The listing builds one solid part. Answer for the finished solid, in the listing's coordinates (mm). Face numbers are marked on the shaded views. A direction names the side the tool comes from. Coordinates: 2 decimals unless noted, no trailing zeros. Write each loop counter-clockwise with the first axis right and the second up, starting at its lowest first coordinate (ties: lowest second). Pieces come first, ordered by that corner, then holes. Notation, with made-up numbers: M -1,-29.75 L 58,-29.75 A17 ccw 58,-19.75 Z; hole C -7.75,34 d5. An arc over 180 degrees is marked long. Answer as CSV lines item,"result". Start each with the question number.
```python
from build123d import *

# Parameters (mm, degrees)
SKETCH1_W           = 60
SKETCH1_H           = 24
BOSS_EXTRUDE1_DEPTH = 3.3
SKETCH2_W           = 3.3
SKETCH2_H           = 24
BOSS_EXTRUDE2_DEPTH = 61.3
SKETCH7_R           = 1.5
SKETCH7_W           = 29.4
SKETCH7_H           = 14
CUT_EXTRUDE4_DEPTH  = 3.3
SKETCH9_W           = 14
SKETCH9_H           = 28
CUT_EXTRUDE5_DEPTH  = 10


with BuildPart() as part:
    # Sketch1 → Boss-Extrude1 (new body)
    with BuildSketch(Plane(origin=(0, 0, 0), x_dir=(1, 0, 0), z_dir=(0, 1, 0))):
        Rectangle(SKETCH1_W, SKETCH1_H)
    extrude(amount=BOSS_EXTRUDE1_DEPTH)

    # Sketch2 → Boss-Extrude2 (add)
    with BuildSketch(Plane(origin=(0, 0, 0), x_dir=(1, 0, 0), z_dir=(0, 1, 0))):
        with Locations((-28.35, 0)):
            Rectangle(SKETCH2_W, SKETCH2_H)
    extrude(amount=BOSS_EXTRUDE2_DEPTH)

    # Sketch7 → Cut-Extrude4 (cut)
    with BuildSketch(Plane(origin=(0, 0, 0), x_dir=(1, 0, 0), z_dir=(0, 1, 0))):
        with Locations((-21.3, 0)):
            Circle(SKETCH7_R)
        with Locations((14.7, 0)):
            Circle(SKETCH7_R)
        with Locations((-3.3, 0)):
            Rectangle(SKETCH7_W, SKETCH7_H)
    extrude(amount=CUT_EXTRUDE4_DEPTH, mode=Mode.SUBTRACT)

    # Sketch9 → Cut-Extrude5 (cut)
    with BuildSketch(Plane.ZY.offset(30)):
        with Locations((-0.012794058, 25)):
            Rectangle(SKETCH9_W, SKETCH9_H)
    extrude(amount=-CUT_EXTRUDE5_DEPTH, mode=Mode.SUBTRACT)


solid = part.part
```
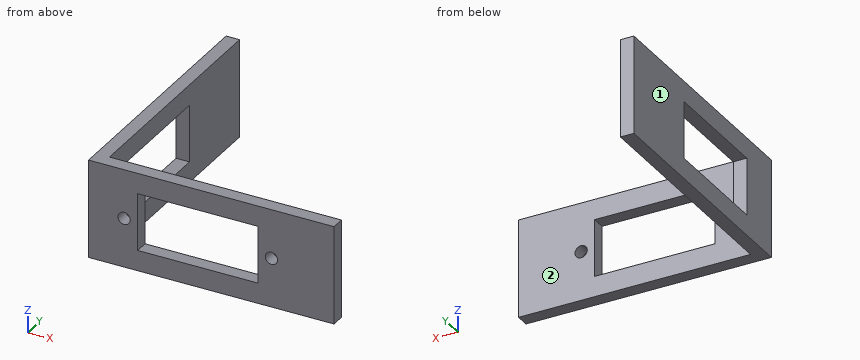
1) Find the intervals of material crossed by line 1 (X direction, y = 2.65, z = 0); line 2 (Z direction, x = -21.3, y = 1.3); line 3 (Y direction, x = -6.5, z = 7.25), in increasing order. Write a range as from..to.
2) Each of these flat-tipped pins is pushed along its axis until it touches: P1, Ø4, axis at x = 14.7, z = 0, coming from the -Y side; P2, Ø12, axis at x = 8.5, z = 4, coming from the +Y side; P3, Ø3, axis at y = 33, z = 7, coming from the +X side. Where does it stop, or does it pass through?
3) The part is cut by section C-C (y = 28). Determine the outline of the cut face in (x, z).
4) The part is cut by section A-A (z = 5). Determine the outline of the cut face in (x, y), then the cut area to 3 significant figures.
5) Which of the six approach directions +Z, -Z, +X, -X, +Y, -Y give full straight-line access (tool end or side, diameter ignored) to the marked faces 1 and 2?
6) The part is cut by section D-D (z = 0). Determine the outline of the cut face in (x, y).
7) The part is cut by section B-B (x = -21.3). Determine the outline of the cut face in (y, z), then the cut area to 3 significant figures.
Completed:
1,line 1,"-30..-22.8, -19.8..-18, 11.4..13.2, 16.2..30"
1,line 2,"-12..-1.5, 1.5..12"
1,line 3,"0..3.3"
2,P1,"y = 0"
2,P2,"y = 3.3"
2,P3,"x = -26.7"
3,outline,"M -30,-12 L -26.7,-12 L -26.7,-7.01 L -30,-7.01 Z; M -30,6.99 L -26.7,6.99 L -26.7,12 L -30,12 Z"
4,outline,"M -30,0 L -18,0 L -18,3.3 L -26.7,3.3 L -26.7,11 L -30,11 Z; M -30,39 L -26.7,39 L -26.7,61.3 L -30,61.3 Z; M 11.4,0 L 30,0 L 30,3.3 L 11.4,3.3 Z"
4,area,"200 mm²"
5,face 1,"+Z, -Z, -X, +Y, -Y"
5,face 2,"+Z, -Z, +X, +Y"
6,outline,"M -30,0 L -22.8,0 L -22.8,3.3 L -26.7,3.3 L -26.7,11 L -30,11 Z; M -30,39 L -26.7,39 L -26.7,61.3 L -30,61.3 Z; M -19.8,0 L -18,0 L -18,3.3 L -19.8,3.3 Z; M 11.4,0 L 13.2,0 L 13.2,3.3 L 11.4,3.3 Z; M 16.2,0 L 30,0 L 30,3.3 L 16.2,3.3 Z"
7,outline,"M 0,-12 L 3.3,-12 L 3.3,-1.5 L 0,-1.5 Z; M 0,1.5 L 3.3,1.5 L 3.3,12 L 0,12 Z"
7,area,"69.3 mm²"
